Build history of the part. All positions in model axes, mm. Face numbers are marked on the shaded views. Coordinates: 2 decimals unless noted, no trailing zeros. Order: outer loops, then holes, each group sorted by start corner. A loop starts at its lowest first (then second) coordinate and runs counter-clockwise, first axis right, second up. Notation, with made-up numbers: (-22.75, 24) - (9.25, 24) arc R29 ccw to (9.25, 56) - close; hole circle Ø3 at (34.25, 62.5). An arc over 180 degrees is marked (long way). One line per item, written item: value.
from build123d import *

# Parameters (mm, degrees)
SKETCH1_R            = 17.5
BOSS_EXTRUDE1_DEPTH  = 10
CHAMFER1_SIZE        = 35
CHAMFER1_EDGE_2_SIZE = 35
CHAMFER1_EDGE_3_SIZE = 35


with BuildPart() as part:
    # Sketch1 → Boss-Extrude1 (new body)
    with BuildSketch(Plane(origin=(0, 0, 0), x_dir=(1, 0, 0), z_dir=(0, 1, 0))):
        Polygon((-5.037101102, -3.128878012), (144.962898898, -3.128878012), (69.962898898, 126.774932556), align=None)
        with Locations(Location((69.962898898, 40.172392178, 0), (0, 0, 270))):
            Circle(SKETCH1_R, mode=Mode.SUBTRACT)
    extrude(amount=BOSS_EXTRUDE1_DEPTH)

    # Chamfer1
    chamfer1_edges = [part.edges().sort_by_distance(p)[0] for p in [
        (69.962898898, 5, -126.774932556),
    ]]
    chamfer(chamfer1_edges, length=CHAMFER1_SIZE)

    # Chamfer1 edge 2
    chamfer1_edge_2_edges = [part.edges().sort_by_distance(p)[0] for p in [
        (144.962898898, 5, 3.128878012),
    ]]
    chamfer(chamfer1_edge_2_edges, length=CHAMFER1_EDGE_2_SIZE)

    # Chamfer1 edge 3
    chamfer1_edge_3_edges = [part.edges().sort_by_distance(p)[0] for p in [
        (-5.037101102, 5, 3.128878012),
    ]]
    chamfer(chamfer1_edge_3_edges, length=CHAMFER1_EDGE_3_SIZE)


solid = part.part
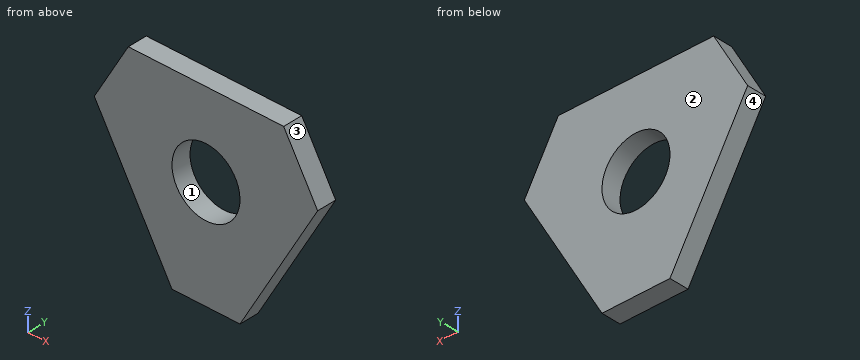
1. Flat gauge pins, fed straight in: P1, Ø5, axis at x = 32, y = 3.5, coming from the -Z side; P2, Ø4, axis at y = 2.5, z = -76.5, coming from the -X side; P3, Ø6, axis at y = 3.5, z = -81, coming from the -X side. Where does each tip first touch, or does it go through?
Values found:
P1: stops at z = -65.35
P2: stops at x = 39.78
P3: stops at x = 41.8
2. Probe line 1 along X through (y, z) = (1, -28); line 2 along X through (y, z) = (7.5, -40.5); line 3 along Z through (x, y) = (55.5, 2). List the from-to ranges inside material, lowest first.
Values found:
line 1: x = 12.94 to 57.39, 82.54 to 126.99
line 2: x = 20.15 to 52.47, 87.46 to 119.77
line 3: z = -96.46 to -50.03, -30.32 to 3.13
3. Band-saw the part on A-A, the plane z = -37. Give the cut face in (x, y), and give its area (3 significant figures).
Values found:
outline: (18.13, 0) - (52.75, 0) - (52.75, 10) - (18.13, 10) - close; (87.17, 0) - (121.79, 0) - (121.79, 10) - (87.17, 10) - close
area: 692 mm2
4. Band-saw the part on B-B, the plane x = 67. Give the cut face in (y, z), and give its area (3 significant figures).
Values found:
outline: (0, -96.46) - (10, -96.46) - (10, -57.42) - (0, -57.42) - close; (0, -22.93) - (10, -22.93) - (10, 3.13) - (0, 3.13) - close
area: 651 mm2
5. Band-saw the part on D-D, the plane z = -60. Give the cut face in (x, y).
Values found:
outline: (31.41, 0) - (108.52, 0) - (108.52, 10) - (31.41, 10) - close
6. Band-saw the part on C-C, the plane y = 5. Give the cut face in (x, z), and give its area (3 significant figures).
Values found:
outline: (12.46, -27.18) - (52.46, -96.46) - (87.46, -96.46) - (127.46, -27.18) - (109.96, 3.13) - (29.96, 3.13) - close; hole circle Ø35 at (69.96, -40.17)
area: 7,190 mm2
7. Two-plate mould, pull along X, no slides. Class the marked faces 1, 2, 3 and 4: pulls with the +X half, pulls with the -X half, needs draft (parallel to the pull), parting line crosses it, or undercut.
Values found:
face 1: undercut
face 2: needs draft
face 3: pulls with the +X half
face 4: pulls with the -X half
